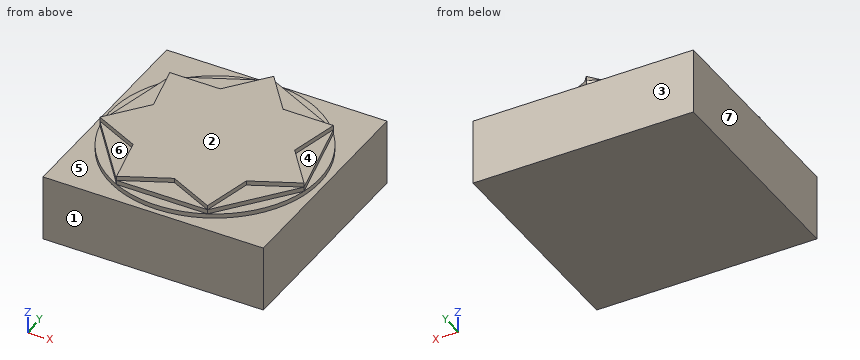
from build123d import *

# Parameters (mm, degrees)
F0_W     = 100
F0_H     = 100
F1_DEPTH = 30
F2_R     = 47.5
F3_DEPTH = 2
F5_DEPTH = 2
F7_DEPTH = 2


# Not quite as in the source:
# - a feature names something its author has since deleted; it is built from what else it names


with BuildPart() as f1:
    # F0 (on Top) → F1 (new body)
    with BuildSketch(Plane.XY):
        Rectangle(F0_W, F0_H)
    extrude(amount=F1_DEPTH)

    # F2 (on face) → F3 (join)
    with BuildSketch(Plane.XY.offset(30)):
        Circle(F2_R)
    extrude(amount=F3_DEPTH)

    # F4 (on face) → F5 (join)
    with BuildSketch(Plane.XY.offset(32)):
        Polygon((37.1369954172, 29.6157655883), (0, 47.5), (-37.1369954172, 29.6157655883), (-46.3090758286, -10.5697443629), (-20.6094776081, -42.7960212254), (20.6094776081, -42.7960212254), (46.3090758286, -10.5697443629), align=None)
    extrude(amount=F5_DEPTH)

    # F6 (on face) → F7 (join)
    with BuildSketch(Plane.XY.offset(34)):
        Polygon((-25.6995982206, -20.4947456859), (-20.6094776081, -42.7960212254), (0, -32.8710199024), (20.6094776081, -42.7960212254), (25.6995982206, -20.4947456859), (46.3090758286, -10.5697443629), (32.0468748048, 7.3144900488), (37.1369954172, 29.6157655883), (14.2622010239, 29.6157655883), (0, 47.5), (-14.2622010239, 29.6157655883), (-37.1369954172, 29.6157655883), (-32.0468748048, 7.3144900488), (-46.3090758286, -10.5697443629), align=None)
    extrude(amount=F7_DEPTH)


solid = f1.part
Read the model definition and answer for the solid it produces. Units are mm, in the model's axes. Face numbers are marked on the shaded views. A direction names the side the tool comes from. Round coordinates to 2 decimals unless told otherwise and drop trailing zeros. Write each loop counter-clockwise with the first axis right and the second up, starting at its lowest first coordinate (ties: lowest second). Pieces come first, ordered by that corner, then holes.
1. Which of the six approach directions +Z, -Z, +X, -X, +Y, -Y give full straight-line access (tool end or side, diameter ignored) to the marked faces 5, 6 and 7?
2. Determine the mould class of the marked faces 1, 2, 3 and 4 for opening direction Y: pulls with the +Y half, pulls with the -Y half, needs draft (parallel to the pull), parting line crosses it, or undercut.
3. Straight lines are drawn through the part: L1, parallel to Z at x = -41, y = 30.5; L2, parallel to Z at x = -12, y = -40; L3, parallel to Y at x = -13, z = 33. For each, find the intervals that lie inside material, in ascending order.
4. Given pin 1 Ø4.5 at (x, y) = (-39.5, 18.5) entering from +Z; pin 2 Ø2 at (x, z) = (-10, 32) entering from +Y; pin 3 Ø1.6 at (x, z) = (-22, 34.5) entering from +Y, each flat-ended and moving along its own axis, determine where each tip first touches the part or whether it passes through.
5. The part is cut by section A-A, the plane x = -17. Determine the outline of the cut face in (y, z).
6. The part is cut by section B-B, the plane y = 34. Determine the outline of the cut face in (x, z).
Values:
1. face 5: +Z
1. face 6: +Z, -X, -Y
1. face 7: +Z, -Z, -X, +Y, -Y
2. face 1: pulls with the -Y half
2. face 2: needs draft
2. face 3: pulls with the +Y half
2. face 4: undercut
3. L1: z = 0 to 30
3. L2: z = 0 to 34
3. L3: y = -42.8 to 41.24
4. pin 1: stops at z = 34
4. pin 2: stops at y = 46.64
4. pin 3: stops at y = 37.21
5. outline: (-50, 0) - (50, 0) - (50, 30) - (44.35, 30) - (44.35, 32) - (39.31, 32) - (39.31, 34) - (29.62, 34) - (29.62, 36) - (-41.06, 36) - (-41.06, 34) - (-42.8, 34) - (-42.8, 32) - (-44.35, 32) - (-44.35, 30) - (-50, 30) - close
6. outline: (-50, 0) - (50, 0) - (50, 30) - (33.17, 30) - (33.17, 32) - (28.03, 32) - (28.03, 34) - (10.77, 34) - (10.77, 36) - (-10.77, 36) - (-10.77, 34) - (-28.03, 34) - (-28.03, 32) - (-33.17, 32) - (-33.17, 30) - (-50, 30) - close
